Could you check a few things on this model? Use its own coordinates, in mm. A direction names the side the tool comes from. Give positions to 0.01 mm unless a question says otherwise; leave off trailing zeros. Order: outer loops, then holes, each group sorted by start corner. A loop starts at its lowest first (then second) coordinate and runs counter-clockwise, first axis right, second up.
from build123d import *

# Parameters (mm, degrees)
SKETCH1_W                = 34
SKETCH1_H                = 30
BOSS_EXTRUDE2_DEPTH      = 51
SKETCH3_R                = 2.55
CUT_EXTRUDE3_DEPTH       = 10
SKETCH5_R                = 7.75
CUT_EXTRUDE4_DEPTH       = 51
SKETCH6_W                = 7
SKETCH6_H                = 30
CUT_EXTRUDE6_DEPTH       = 51
CUT_EXTRUDE7_DEPTH       = 51
CUT_EXTRUDE9_DEPTH       = 1.5
CUT_EXTRUDE9_DEPTH_BACK  = 1.5
BOSS_EXTRUDE5_DEPTH      = 51
CUT_EXTRUDE10_DEPTH      = 13
CUT_EXTRUDE11_DEPTH      = 13
SKETCH13_W               = 2
SKETCH13_H               = 6
CUT_EXTRUDE12_DEPTH      = 2
CUT_EXTRUDE13_DEPTH      = 13
CUT_EXTRUDE13_DEPTH_BACK = 11
BOSS_EXTRUDE6_DEPTH      = 2.25
BOSS_EXTRUDE7_DEPTH      = 2.25
BOSS_EXTRUDE8_DEPTH      = 2.25
BOSS_EXTRUDE9_DEPTH      = 2.25
SKETCH22_W               = 5
SKETCH22_H               = 6
BOSS_EXTRUDE10_DEPTH     = 1
SKETCH24_W               = 5
SKETCH24_H               = 6
BOSS_EXTRUDE11_DEPTH     = 1
SKETCH25_R               = 0.6
CUT_EXTRUDE14_DEPTH      = 20
SKETCH26_R               = 2.55
BOSS_EXTRUDE12_DEPTH     = 1.5
CUT_EXTRUDE16_DEPTH      = 60


with BuildPart() as part:
    # Sketch1 → Boss-Extrude2 (new body)
    with BuildSketch(Plane(origin=(0, 0, 0), x_dir=(0, 0, -1), z_dir=(1, 0, 0))):
        with Locations((-3.945183, 6.145902)):
            Rectangle(SKETCH1_W, SKETCH1_H)
    extrude(amount=BOSS_EXTRUDE2_DEPTH)

    # Sketch3 → Cut-Extrude3 (cut)
    with BuildSketch(Plane(origin=(0, 0, -13.054817), x_dir=(-1, 0, 0), z_dir=(0, 0, -1))):
        with Locations((-25.5, -1.354098)):
            Circle(SKETCH3_R)
    extrude(amount=-CUT_EXTRUDE3_DEPTH, mode=Mode.SUBTRACT)

    # Sketch5 → Cut-Extrude4 (cut)
    with BuildSketch(Plane(origin=(51, 0, 0), x_dir=(0, 0, -1), z_dir=(1, 0, 0))):
        with Locations((-3.945183, 1.145902)):
            Circle(SKETCH5_R)
    extrude(amount=-CUT_EXTRUDE4_DEPTH, mode=Mode.SUBTRACT)

    # Sketch6 → Cut-Extrude6 (cut)
    with BuildSketch(Plane(origin=(51, 0, 0), x_dir=(0, 0, -1), z_dir=(1, 0, 0))):
        with Locations((9.554817, 6.145902)):
            Rectangle(SKETCH6_W, SKETCH6_H)
    extrude(amount=-CUT_EXTRUDE6_DEPTH, mode=Mode.SUBTRACT)

    # Sketch7 → Cut-Extrude7 (cut)
    with BuildSketch(Plane(origin=(51, 0, 0), x_dir=(0, 0, -1), z_dir=(1, 0, 0))):
        with BuildLine():
            Line((-3.945183, -8.854098), (-20.945183, -8.854098))
            Line((-20.945183, -8.854098), (-20.945183, 21.145902))
            Line((-20.945183, 21.145902), (6.054817, 21.145902))
            Line((6.054817, 21.145902), (6.054817, 1.145902))
            ThreePointArc((6.054817, 1.145902), (-11.016251, 8.21697), (-3.945183, -8.854098))
        make_face()
    extrude(amount=-CUT_EXTRUDE7_DEPTH, mode=Mode.SUBTRACT)

    # Sketch8 → Cut-Extrude9 (cut, two sides)
    with BuildSketch(Plane(origin=(0, 0, -3.054817), x_dir=(-1, 0, 0), z_dir=(0, 0, -1))) as cut_extrude9_sk:
        Polygon((-21.75, -2.180132), (-21.75, -4.904098), (-29.25, -4.904098), (-29.25, -2.180132), (-29.25, 2.195902), (-21.75, 2.195902), align=None)
    extrude(amount=CUT_EXTRUDE9_DEPTH, mode=Mode.SUBTRACT)
    extrude(cut_extrude9_sk.sketch, amount=-CUT_EXTRUDE9_DEPTH_BACK, mode=Mode.SUBTRACT)

    # Sketch10 → Boss-Extrude5 (add)
    with BuildSketch(Plane(origin=(51, 0, 0), x_dir=(0, 0, -1), z_dir=(1, 0, 0))):
        Polygon((-17.695183, 1.145902), (-17.695183, 4.145902), (-11.695183, 4.145902), (-11.695183, 1.145902), (-11.695183, -1.854098), (-17.695183, -1.854098), align=None)
    extrude(amount=-BOSS_EXTRUDE5_DEPTH)

    # Sketch11 → Cut-Extrude10 (cut)
    with BuildSketch(Plane(origin=(51, 0, 0), x_dir=(0, 0, -1), z_dir=(1, 0, 0))):
        with BuildLine():
            Line((-13.484575, -1.854098), (-17.695183, -1.854098))
            Line((-17.695183, -1.854098), (-17.695183, 4.145902))
            Line((-17.695183, 4.145902), (-13.484575, 4.145902))
            ThreePointArc((-13.484575, 4.145902), (-13.945183, 1.145902), (-13.484575, -1.854098))
        make_face()
    extrude(amount=-CUT_EXTRUDE10_DEPTH, mode=Mode.SUBTRACT)

    # Sketch12 → Cut-Extrude11 (cut)
    with BuildSketch(Plane.ZY):
        with BuildLine():
            Line((13.484575, -1.854098), (17.695183, -1.854098))
            Line((17.695183, -1.854098), (17.695183, 4.145902))
            Line((17.695183, 4.145902), (13.484575, 4.145902))
            ThreePointArc((13.484575, 4.145902), (13.945183, 1.145902), (13.484575, -1.854098))
        make_face()
    extrude(amount=-CUT_EXTRUDE11_DEPTH, mode=Mode.SUBTRACT)

    # Sketch13 → Cut-Extrude12 (cut)
    with BuildSketch(Plane.XY.offset(17.695183)):
        with Locations((25.5, 1.145902)):
            Rectangle(SKETCH13_W, SKETCH13_H)
    extrude(amount=-CUT_EXTRUDE12_DEPTH, mode=Mode.SUBTRACT)

    # Sketch15 → Cut-Extrude13 (cut, two sides)
    with BuildSketch(Plane(origin=(24.5, 0, 0), x_dir=(0, 0, -1), z_dir=(1, 0, 0))) as cut_extrude13_sk:
        with BuildLine():
            Line((-17.695183, 4.145902), (-17.695183, -1.854098))
            Line((-17.695183, -1.854098), (-13.484575, -1.854098))
            ThreePointArc((-13.484575, -1.854098), (-13.945183, 1.145902), (-13.484575, 4.145902))
            Line((-13.484575, 4.145902), (-17.695183, 4.145902))
        make_face()
    extrude(amount=CUT_EXTRUDE13_DEPTH, mode=Mode.SUBTRACT)
    extrude(cut_extrude13_sk.sketch, amount=-CUT_EXTRUDE13_DEPTH_BACK, mode=Mode.SUBTRACT)

    # Sketch17 → Boss-Extrude6 (add)
    with BuildSketch(Plane(origin=(38, 0, 0), x_dir=(0, 0, -1), z_dir=(1, 0, 0))):
        with BuildLine():
            Line((-13.484575, 4.145902), (-17.695183, 4.145902))
            Line((-17.695183, 4.145902), (-17.695183, -1.854098))
            Line((-17.695183, -1.854098), (-13.484575, -1.854098))
            ThreePointArc((-13.484575, -1.854098), (-13.945183, 1.145902), (-13.484575, 4.145902))
        make_face()
    extrude(amount=BOSS_EXTRUDE6_DEPTH)

    # Sketch19 → Boss-Extrude7 (add)
    with BuildSketch(Plane.ZY.offset(-13)):
        with BuildLine():
            Line((13.484575, 4.145902), (17.695183, 4.145902))
            Line((17.695183, 4.145902), (17.695183, -1.854098))
            Line((17.695183, -1.854098), (13.484575, -1.854098))
            ThreePointArc((13.484575, -1.854098), (13.945183, 1.145902), (13.484575, 4.145902))
        make_face()
    extrude(amount=BOSS_EXTRUDE7_DEPTH)

    # Sketch20 → Boss-Extrude8 (add)
    with BuildSketch(Plane(origin=(13.5, 0, 0), x_dir=(0, 0, -1), z_dir=(1, 0, 0))):
        with BuildLine():
            Line((-17.695183, -1.854098), (-17.695183, 4.145902))
            Line((-17.695183, 4.145902), (-13.484575, 4.145902))
            ThreePointArc((-13.484575, 4.145902), (-13.945183, 1.145902), (-13.484575, -1.854098))
            Line((-13.484575, -1.854098), (-17.695183, -1.854098))
        make_face()
    extrude(amount=BOSS_EXTRUDE8_DEPTH)

    # Sketch21 → Boss-Extrude9 (add)
    with BuildSketch(Plane.ZY.offset(-37.5)):
        with BuildLine():
            Line((13.484575, 4.145902), (17.695183, 4.145902))
            Line((17.695183, 4.145902), (17.695183, -1.854098))
            Line((17.695183, -1.854098), (13.484575, -1.854098))
            ThreePointArc((13.484575, -1.854098), (13.945183, 1.145902), (13.484575, 4.145902))
        make_face()
    extrude(amount=BOSS_EXTRUDE9_DEPTH)

    # Sketch22 → Boss-Extrude10 (add)
    with BuildSketch(Plane.XY.offset(17.695183)):
        with Locations((37.75, 1.145902)):
            Rectangle(SKETCH22_W, SKETCH22_H)
    extrude(amount=BOSS_EXTRUDE10_DEPTH)

    # Sketch24 → Boss-Extrude11 (add)
    with BuildSketch(Plane.XY.offset(17.695183)):
        with Locations((13.25, 1.145902)):
            Rectangle(SKETCH24_W, SKETCH24_H)
    extrude(amount=BOSS_EXTRUDE11_DEPTH)

    # Sketch25 → Cut-Extrude14 (cut)
    with BuildSketch(Plane(origin=(0, 4.145902, 0), x_dir=(1, 0, 0), z_dir=(0, 1, 0))):
        with Locations((13.25, -16.695183)):
            Circle(SKETCH25_R)
        with Locations((37.75, -16.695183)):
            Circle(SKETCH25_R)
    extrude(amount=-CUT_EXTRUDE14_DEPTH, mode=Mode.SUBTRACT)

    # Sketch26 → Boss-Extrude12 (add)
    with BuildSketch(Plane(origin=(0, 0, -6.054817), x_dir=(-1, 0, 0), z_dir=(0, 0, -1))):
        with Locations((-25.5, -1.354098)):
            Circle(SKETCH26_R)
    extrude(amount=-BOSS_EXTRUDE12_DEPTH)

    # Sketch27 → Cut-Extrude16 (cut)
    with BuildSketch(Plane(origin=(51, 0, 0), x_dir=(0, 0, -1), z_dir=(1, 0, 0))):
        Polygon((-18.695183, 1.145902), (-18.695183, 12.015935), (6.594767, 12.015935), (6.594767, 1.145902), (6.594767, 0.645902), (-18.695183, 0.645902), align=None)
    extrude(amount=-CUT_EXTRUDE16_DEPTH, mode=Mode.SUBTRACT)


solid = part.part
Item 1: Imagine slicing it at B-B on x = 13.25. List the corners of the cut face in (y, z) for me.
Findings:
outline: (-8.85, -6.05) - (0.65, -6.05) - (0.65, -3.79) arc R7.75 cw to (0.65, 11.68) - (0.65, 16.1) - (-1.85, 16.1) - (-1.85, 13.48) arc R10 ccw to (-8.85, 3.95) - close; (-1.85, 17.3) - (0.65, 17.3) - (0.65, 18.7) - (-1.85, 18.7) - close
Item 2: We'd pull the mould along Z, two halves only. Please class faces 1 (the cylindrical face through (13.17, -0.59, 16.1)), 2 (the flat face through (10.75, -1, 16)), 3 (the flat face through (38, -1, 18.695)): +Z half, -Z half, draft (parallel to the pull), parting line (faces both ways), or undercut.
Findings:
face 1: undercut
face 2: draft
face 3: +Z half
Item 3: Imagine slicing it at D-D on x = 23. List the corners of the cut face in (y, z) for me, then the cut area to 3 significant figures.
Findings:
outline: (-8.85, -6.05) - (0.65, -6.05) - (0.65, -4.55) - (-4.9, -4.55) - (-4.9, -1.55) - (-4.31, -1.55) arc R7.75 cw to (0.65, 11.68) - (0.65, 13.93) arc R10 ccw to (-8.85, 3.95) - close
area: 72.6 mm2
Item 4: For pin 1 (0.9 mm diameter, centred on y = -1, z = -3, fed in from +X); pin 2 (4 mm diameter, centred on x = 29, z = 9, fed in from +Y); pin 3 (1.5 mm diameter, centred on x = 37, z = 16.5, fed in from -Y); pin 4 (0.8 mm diameter, centred on y = -1, z = 16, fed in from +X), each with a flat end and sliding along its axis, tell me the tip position at first contact or that it passes through.
Findings:
pin 1: passes through
pin 2: stops at y = -2.06
pin 3: stops at y = -1.85
pin 4: stops at x = 40.25
Item 5: Imagine slicing it at A-A on z = 15.5. List the corners of the cut face in (x, y) for me.
Findings:
outline: (10.75, -1.85) - (15.75, -1.85) - (15.75, 0.65) - (10.75, 0.65) - close; (35.25, -1.85) - (40.25, -1.85) - (40.25, 0.65) - (35.25, 0.65) - close
Item 6: For faces 4 (the flat face through (0, -7, 2)), 5 (the flat face through (38, -1.854, 15)), 6 (the flat face through (25, -2, -4.555)), which set-ups out of +Z, -Z, +X, -X, +Y, -Y let a thin tool reach every point of the face, with its end or its side?
Findings:
face 4: +Z, -Z, -X, +Y, -Y
face 5: +Z, +X, -X, -Y
face 6: +Y
Item 7: Imagine slicing it at C-C on y = -1.25. List the corners of the cut face in (x, z) for me.
Findings:
outline: (0, -6.05) - (51, -6.05) - (51, -3.43) - (29.25, -3.43) - (29.25, -4.55) - (21.75, -4.55) - (21.75, -3.43) - (0, -3.43) - close; (0, 11.32) - (51, 11.32) - (51, 13.65) - (40.25, 13.65) - (40.25, 18.7) - (35.25, 18.7) - (35.25, 13.65) - (15.75, 13.65) - (15.75, 18.7) - (10.75, 18.7) - (10.75, 13.65) - (0, 13.65) - close; hole circle Ø1.2 at (13.25, 16.7); hole circle Ø1.2 at (37.75, 16.7)
Item 8: Please list where these lines run through material, in increasing order: line 1 along X through (y, z) = (-2.5, -4.25); line 2 along Z through (x, y) = (13.25, -0.2); line 3 along Z through (x, y) = (37.75, -1.1).
Findings:
line 1: x = 0 to 21.75, 29.25 to 51
line 2: z = -6.05 to -3.69, 11.58 to 16.1, 17.3 to 18.7
line 3: z = -6.05 to -3.47, 11.36 to 16.1, 17.3 to 18.7
